from build123d import *

# Parameters (mm, degrees)
SKETCH_1_R          = 16.25
EXTRUDE_1_DEPTH     = 27
SHELL_1_T           = -2
SKETCH_2_R          = 6.75
SKETCH_2_R_2        = 1.65
CUT_EXTRUDE_1_DEPTH = 27
SKETCH_3_R          = 23
SKETCH_3_R_2        = 14.25
SKETCH_3_R_3        = 1.65
EXTRUDE_2_DEPTH     = 3


with BuildPart() as part:
    # 草图1 → 凸台-拉伸1 (new body)
    with BuildSketch(Plane(origin=(0, 0, 0), x_dir=(1, 0, 0), z_dir=(0, 1, 0))):
        with Locations(Location((0, 0, 0), (0, 0, 270))):
            Circle(SKETCH_1_R)
    extrude(amount=EXTRUDE_1_DEPTH)

    # 抽壳1
    shell_1_openings = [part.faces().sort_by_distance(p)[0] for p in [
        (0, 27, 0),
    ]]
    offset(amount=SHELL_1_T, openings=shell_1_openings, kind=Kind.INTERSECTION)

    # 草图2 → 切除-拉伸1 (cut)
    with BuildSketch(Plane.XZ):
        with Locations(Location((0, 0, 0), (0, 0, 270))):
            Circle(SKETCH_2_R)
        with Locations(Location((4.75, 8.227241336, 0), (0, 0, 270))):
            Circle(SKETCH_2_R_2)
        with Locations(Location((9.5, 0, 0), (0, 0, 270))):
            Circle(SKETCH_2_R_2)
        with Locations(Location((4.75, -8.227241336, 0), (0, 0, 270))):
            Circle(SKETCH_2_R_2)
        with Locations(Location((-4.75, -8.227241336, 0), (0, 0, 270))):
            Circle(SKETCH_2_R_2)
        with Locations(Location((-9.5, 0, 0), (0, 0, 270))):
            Circle(SKETCH_2_R_2)
        with Locations(Location((-4.75, 8.227241336, 0), (0, 0, 270))):
            Circle(SKETCH_2_R_2)
    extrude(amount=-CUT_EXTRUDE_1_DEPTH, mode=Mode.SUBTRACT)

    # 草图3 → 凸台-拉伸2 (add)
    with BuildSketch(Plane(origin=(0, 27, 0), x_dir=(1, 0, 0), z_dir=(0, 1, 0))):
        with Locations(Location((0, 0, 0), (0, 0, 270))):
            Circle(SKETCH_3_R)
        with Locations(Location((0, 0, 0), (0, 0, 270))):
            Circle(SKETCH_3_R_2, mode=Mode.SUBTRACT)
        with Locations(Location((0, 20, 0), (0, 0, 270))):
            Circle(SKETCH_3_R_3, mode=Mode.SUBTRACT)
        with Locations(Location((17.320508076, 10, 0), (0, 0, 270))):
            Circle(SKETCH_3_R_3, mode=Mode.SUBTRACT)
        with Locations(Location((17.320508076, -10, 0), (0, 0, 270))):
            Circle(SKETCH_3_R_3, mode=Mode.SUBTRACT)
        with Locations(Location((0, -20, 0), (0, 0, 270))):
            Circle(SKETCH_3_R_3, mode=Mode.SUBTRACT)
        with Locations(Location((-17.320508076, -10, 0), (0, 0, 270))):
            Circle(SKETCH_3_R_3, mode=Mode.SUBTRACT)
        with Locations(Location((-17.320508076, 10, 0), (0, 0, 270))):
            Circle(SKETCH_3_R_3, mode=Mode.SUBTRACT)
    extrude(amount=EXTRUDE_2_DEPTH)


solid = part.part
Model file for the job. Use its own axes, mm. A direction names the side the tool comes from. Round coordinates to 2 decimals unless told otherwise and drop trailing zeros. Loops run counter-clockwise (first coordinate to the right, second up) from the corner with the lowest first, then second, coordinate; pieces in that order, holes last. Notation, with made-up numbers: (24.5, 41) - (61.5, 41) arc R20 cw to (61.5, 46) - close; hole circle Ø9 at (8, 12). An arc over 180 degrees is marked (long way). Write each question's results on one line, items separated by ' | '.
(1) 3-axis set-ups, long thin cutter, end or side, ignore diameter. For faces 1 (the flat face through (16, 27, 5)), 2 (the cylindrical face through (-13.91, 15.8, -3.09)), 3 (the cylindrical face through (4.118, 0.986, -9.751)): which of +Z, -Z, +X, -X, +Y, -Y reach the whole face in a straight line?
Answer below:
face 1: -Y | face 2: +Y | face 3: +Y, -Y
(2) Wall check: L1, parallel to X at y = 6, z = 0; L2, parallel to Y at x = -3.5, z = -17; L3, parallel to X at y = 28.05, z = -10. Give the ranges that are in metal, low to high.
Answer below:
L1: x = -16.25 to -14.25, 14.25 to 16.25 | L2: y = 27 to 30 | L3: x = -20.71 to -18.97, -15.67 to -10.15, 10.15 to 15.67, 18.97 to 20.71
(3) Pin check, flat tips, straight feed: pin 1 (2 mm diameter, centred on y = 25.5, z = 16, fed in from -X); pin 2 (2 mm diameter, centred on x = 14, y = 7, fed in from -Z); pin 3 (1 mm diameter, centred on x = -0.5, z = 14.5, fed in from -Y); pin 4 (6 mm diameter, centred on x = -7, z = -7.5, fed in from +Y). Stop position of each tip, or through.
Answer below:
pin 1: stops at x = -6.25 | pin 2: stops at z = -9.75 | pin 3: stops at y = 0 | pin 4: stops at y = 2
(4) Saw through at D-D, the plane y = 24. List the corners of the cut face in (x, z), then the cut area to 3 significant figures.
Answer below:
outline: circle Ø32.5 at (0, 0); hole circle Ø28.5 at (0, 0) | area: 192 mm^2
(5) Saw through at A-A, the plane x = 0. List the corners of the cut face in (y, z), then the cut area to 3 significant figures.
Answer below:
outline: (0, -16.25) - (27, -16.25) - (27, -18.35) - (30, -18.35) - (30, -14.25) - (2, -14.25) - (2, -6.75) - (0, -6.75) - close; (0, 6.75) - (2, 6.75) - (2, 14.25) - (30, 14.25) - (30, 18.35) - (27, 18.35) - (27, 16.25) - (0, 16.25) - close; (27, -23) - (30, -23) - (30, -21.65) - (27, -21.65) - close; (27, 21.65) - (30, 21.65) - (30, 23) - (27, 23) - close | area: 171 mm^2
(6) Mould opens along X. For faces 4 (the cylindrical face through (-1, 28.48, -21.31)), 5 (the flat face through (-10, 30, -11)), 6 (the cylindrical face through (4.88, 13.31, 15.5)) say: released by +X, released by -X, zero draft, split by the parting line, or undercut.
Answer below:
face 4: undercut | face 5: zero draft | face 6: split by the parting line
(7) Saw through at C-C, the plane x = 9.5. List the corners of the cut face in (y, z).
Answer below:
outline: (0, -13.18) - (27, -13.18) - (27, -20.95) - (30, -20.95) - (30, -10.62) - (2, -10.62) - (2, -1.65) - (0, -1.65) - close; (0, 1.65) - (2, 1.65) - (2, 10.62) - (30, 10.62) - (30, 20.95) - (27, 20.95) - (27, 13.18) - (0, 13.18) - close
(8) Saw through at B-B, the plane z = 1. List the corners of the cut face in (x, y).
Answer below:
outline: (-22.98, 27) - (-16.22, 27) - (-16.22, 0) - (-10.81, 0) - (-10.81, 2) - (-14.21, 2) - (-14.21, 30) - (-22.98, 30) - close; (-8.19, 0) - (-6.68, 0) - (-6.68, 2) - (-8.19, 2) - close; (6.68, 0) - (8.19, 0) - (8.19, 2) - (6.68, 2) - close; (10.81, 0) - (16.22, 0) - (16.22, 27) - (22.98, 27) - (22.98, 30) - (14.21, 30) - (14.21, 2) - (10.81, 2) - close
